Source: CAD feature listing. Evaluate the final solid. Frame: model axes, mm. A direction names the side the tool comes from. Round coordinates to 2 decimals unless told otherwise and drop trailing zeros. Write each loop counter-clockwise with the first axis right and the second up, starting at its lowest first coordinate (ties: lowest second). Pieces come first, ordered by that corner, then holes.
from build123d import *

# Parameters (mm, degrees)
SKETCH1_W          = 95.25
SKETCH1_H          = 87.376
SKETCH1_R          = 34.1503
EXTRUDE1_DEPTH     = 57.15
CUT_EXTRUDE1_DEPTH = 96.25
SKETCH3_R          = 36.576
CUT_EXTRUDE2_DEPTH = 41.275
FILLET1_R          = 1.524
HOLE1_D            = 7.1374
HOLE1_DEPTH        = 87.376


with BuildPart() as part:
    # Sketch1 → Extrude1 (new body)
    with BuildSketch(Plane.XY):
        with Locations((0, 43.688)):
            Rectangle(SKETCH1_W, SKETCH1_H)
        with Locations((0, 44.45)):
            Circle(SKETCH1_R, mode=Mode.SUBTRACT)
    extrude(amount=-EXTRUDE1_DEPTH)

    # Sketch2 → Cut-Extrude1 (cut, through all)
    with BuildSketch(Plane(origin=(47.625, 0, 0), x_dir=(0, 0, -1), z_dir=(1, 0, 0))):
        Polygon((19.05, 87.376), (57.15, 21.336), (57.15, 87.376), align=None)
    extrude(amount=-CUT_EXTRUDE1_DEPTH, mode=Mode.SUBTRACT)

    # Sketch3 → Cut-Extrude2 (cut)
    with BuildSketch(Plane(origin=(0, 0, -57.15), x_dir=(-1, 0, 0), z_dir=(0, 0, -1))):
        with Locations(Location((0, 44.45, 0), (0, 0, 320.806273741))):  # turned: the seam where the file's is
            Circle(SKETCH3_R)
    extrude(amount=-CUT_EXTRUDE2_DEPTH, mode=Mode.SUBTRACT)

    # Fillet1
    fillet1_edges = [part.edges().sort_by_distance(p)[0] for p in [
        (28.346900713, 67.564, -15.875),
    ]]
    fillet(fillet1_edges, radius=FILLET1_R)

    # Hole1
    with Locations(Plane(origin=(0, 87.376, 0), x_dir=(-1, 0, 0), z_dir=(0, 1, 0))):
        with Locations((41.275, -7.874), (-41.275, -7.874)):
            Hole(HOLE1_D / 2, depth=HOLE1_DEPTH)


solid = part.part
1) Section query A-A on y = 44.45. Return the cut outline in (x, z) (3 decimals), then the cut area to 3 significant figures.
Taken from the geometry:
outline: (-47.625, -43.815) - (-36.576, -43.815) - (-36.576, -17.399) arc R1.524 cw to (-35.052, -15.875) - (-34.15, -15.875) - (-34.15, 0) - (-47.625, 0) - close; (34.15, -15.875) - (35.052, -15.875) arc R1.524 cw to (36.576, -17.399) - (36.576, -43.815) - (47.625, -43.815) - (47.625, 0) - (34.15, 0) - close; hole circle Ø7.137 at (-41.275, -7.874); hole circle Ø7.137 at (41.275, -7.874)
area: 966 mm2
2) Pull-direction query (Y, two-part tool) for faces 3 (the face through (-7.4, 11.11, -7.83)), 4 (the face through (20, 15, 0)), 5 (the face through (-1, 87.376, -9)); classes: released by +Y, released by -Y, zero draft, split by the parting line, or undercut.
Taken from the geometry:
face 3: undercut
face 4: zero draft
face 5: released by +Y
3) Contact query for flat-ended pins moving along their axis: P1, Ø3, axis at x = -13.5, z = -26, coming from the +Y side; P2, Ø6.5, axis at x = -41.275, z = -7.874, coming from the +Y side. Output: stop coordinate, or through.
Taken from the geometry:
P1: stops at y = 11.09
P2: passes through
4) Section query B-B on x = 0. Return the cut outline in (y, z) (3 decimals).
Taken from the geometry:
outline: (0, -57.15) - (7.874, -57.15) - (7.874, -17.399) arc R1.524 cw to (9.398, -15.875) - (10.3, -15.875) - (10.3, 0) - (0, 0) - close; (78.6, -15.875) - (79.502, -15.875) arc R1.524 cw to (81.026, -17.399) - (81.026, -22.713) - (87.376, -19.05) - (87.376, 0) - (78.6, 0) - close
5) Section query D-D on y = 63. State how many separate pieces and enclosed holes the cut face has, then the cut area to 3 significant figures.
Taken from the geometry:
separate pieces: 2
enclosed holes: 2
area: 1,080 mm2
6) Reachability of faces 1 (the face through (15.3, 13.6, -15.875)), 2 (the face through (43.194, 43.076, -4.865)) from +Z, -Z, +X, -X, +Y, -Y: full face, straight path, thin tool, end or side. Return the list, or none.
Taken from the geometry:
face 1: -Z
face 2: +Y, -Y
7) Material intervals for line 1 (Y direction, x = 0, z = -10); line 2 (X direction, y = 44, z = -7) (3 decimals); line 3 (Z direction, x = -24.5, y = 68.5) (3 decimals), sorted ascending.
Taken from the geometry:
line 1: y = 0 to 10.3, 78.6 to 87.38
line 2: x = -47.625 to -44.735, -37.815 to -34.147, 34.147 to 37.815, 44.735 to 47.625
line 3: z = -15.875 to 0
8) Section query C-C on z = -40. Return the cut outline in (x, y) (3 decimals), then the cut area to 3 significant figures.
Taken from the geometry:
outline: (-47.625, 0) - (47.625, 0) - (47.625, 51.063) - (35.973, 51.063) arc R36.576 cw (long way) to (-35.973, 51.063) - (-47.625, 51.063) - close
area: 2,280 mm2
